Design review of the part built by this model. Coordinates are the model's own, in mm. A direction names the side the tool comes from. Coordinates: 2 decimals unless noted, no trailing zeros. Loops run counter-clockwise (first coordinate to the right, second up) from the corner with the lowest first, then second, coordinate; pieces in that order, holes last. Notation, with made-up numbers: (-13, -34) - (31, -34) arc R21 ccw to (31, -15) - close; hole circle Ø9 at (-25.5, 18.25). An arc over 180 degrees is marked (long way). Answer in a Markdown table with one row per item. Add a question column.
(1) We need section B-B, the plane x = -22. Write out the cut boundary in (y, z), plus the area to 3 significant figures.
(2) We need section A-A, the plane y = 60.5. Write out the cut boundary in (x, z).
(3) To check wall thickness, follow L1, parallel to Z at x = 29.5, y = 74; L2, parallel to X at y = 90, z = 1.25; L3, parallel to Y at x = 2.5, z = 6.5. State the ranges of each line that lie inside material, in increasing order. Write a range as [from, to].
(4) The part is to be moulded in two halves that separate along Z. For faces 4 (the face through (12.76, 108, 4)), 5 (the face through (2.6, 108, 4)), 6 (the face through (-26.904, 11.503, 0.69)), 7 (the face through (8, 108, 7.6)), say which applies: released by +Z, released by -Z, zero draft, split by the parting line, or undercut.
(5) For faces 1 (the face through (8, 105.708, 4)), 2 (the face through (8, 109.772, 4)), 3 (the face through (7, 50, 0)), list the 3-axis set-ups (+Z, -Z, +X, -X, +Y, -Y) from which the entire face can be reached by the end or side of a thin tool; tool diameter is ignored.
(6) Clearance check with flat-ended pins moving along their axes: pin 1 (4 mm diameter, centred on y = 107.5, z = 5.5, fed in from +X); pin 2 (1 mm diameter, centred on x = 7, z = 7, fed in from +Y); pin 3 (1.1 mm diameter, centred on y = 89, z = 1, fed in from -X). State where each tip first meets the part, or that it passes through.
from build123d import *

# Parameters (mm, degrees)
F1_DEPTH = 1.4
F2_W     = 10.16
F2_H     = 4.064
F3_DEPTH = 5
F4_W     = 12.76
F4_H     = 6.664
F5_DEPTH = 1.2


with BuildPart() as f1:
    # F0 (on Top) → F1 (new body)
    with BuildSketch(Plane.XY):
        Polygon((-39.320156, -3.294921), (-39.320156, -13.294921), (54.679844, -13.294921), (54.679844, -3.294921), (30.189636, 25.891372), (30.189636, 115.891372), (7.679844, 145.469573), (-14.829948, 115.891372), (-14.829948, 25.891372), align=None)
    extrude(amount=F1_DEPTH)

    # F2 (on face) → F3 (join)
    with BuildSketch(Plane.XY.offset(1.4)):
        with Locations((7.679844, 107.740323)):
            Rectangle(F2_W, F2_H)
    extrude(amount=F3_DEPTH)

    # F4 (on face) → F5 (join)
    with BuildSketch(Plane.XY.offset(6.4)):
        with Locations((7.679844, 107.740323)):
            Rectangle(F4_W, F4_H)
    extrude(amount=F5_DEPTH)


solid = f1.part
Responses:
| question | item | result |
|---|---|---|
| 1 | outline | (-13.29, 0) - (17.35, 0) - (17.35, 1.4) - (-13.29, 1.4) - close |
| 1 | area | 42.9 mm2 |
| 2 | outline | (-14.83, 0) - (30.19, 0) - (30.19, 1.4) - (-14.83, 1.4) - close |
| 3 | L1 | z = [0, 1.4] |
| 3 | L2 | x = [-14.83, 30.19] |
| 3 | L3 | y = [104.41, 111.07] |
| 4 | face 4 | undercut |
| 4 | face 5 | undercut |
| 4 | face 6 | zero draft |
| 4 | face 7 | released by +Z |
| 5 | face 1 | +X, -X, -Y |
| 5 | face 2 | +X, -X, +Y |
| 5 | face 3 | -Z, +X, -X, +Y, -Y |
| 6 | pin 1 | stops at x = 14.06 |
| 6 | pin 2 | stops at y = 111.07 |
| 6 | pin 3 | stops at x = -14.83 |
